Print and shaded views of the part. All mm, measured from the part's lowest x, y and z. Give positions to 0.01 mm unless a question says otherwise; leave off trailing zeros. Loops run counter-clockwise (first coordinate to the right, second up) from the corner with the lowest first, then second, coordinate; pieces in that order, holes last. Notation, with made-up numbers: (-3.75, 76) -> (16.25, 76) arc R19 ccw to (16.25, 82) -> close; hole circle Ø7 at (61.5, 52). An arc over 180 degrees is marked (long way). Answer as a JSON object with one key per item and string values. Group by question number.
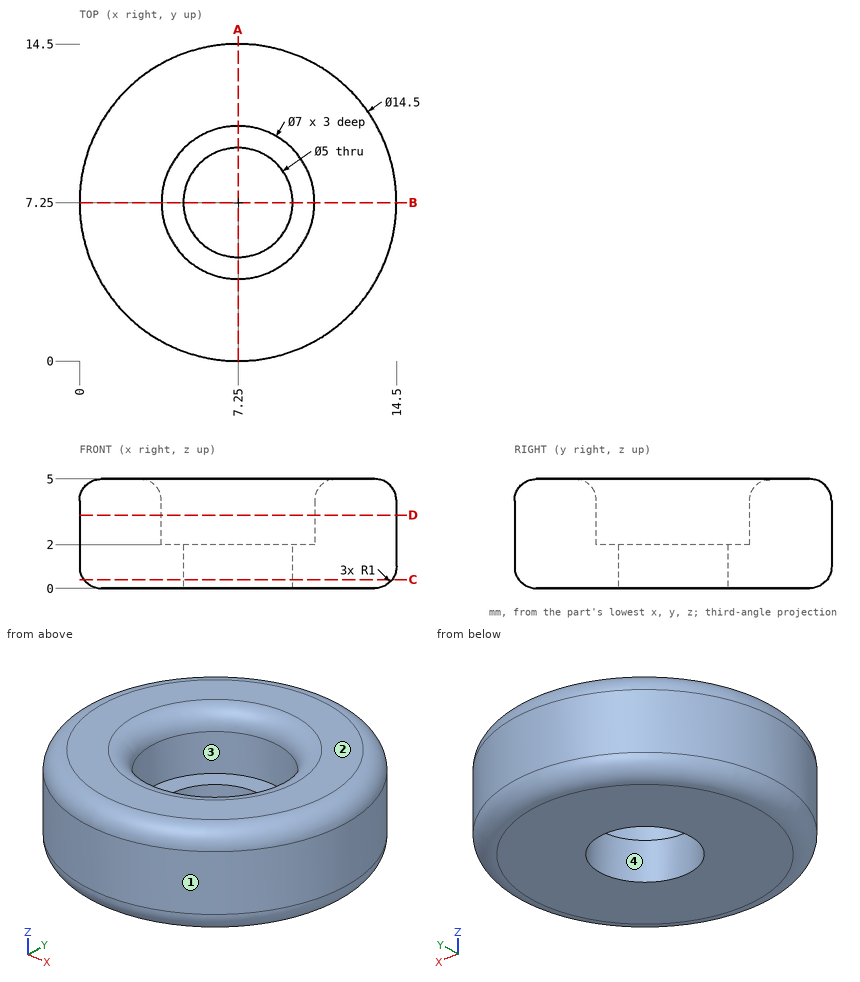
(1) Saw through at C-C on z = 0.4. List the corners of the cut face in (x, y).
(2) Saw through at A-A on x = 7.25. List the corners of the cut face in (y, z), plus the area to 3 significant figures.
(3) Probe line 1 along Y through (x, z) = (7.25, 2.95); line 2 along Z through (x, y) = (8.75, 9.75); line 3 along Y through (x, z) = (7, 0.75). List the from-to ranges inside material, lowest first. Write a range as [from, to].
(4) Saw through at D-D on z = 3.35. List the corners of the cut face in (x, y), plus the area to 3 significant figures.
(5) Pull direction Y, two halves, no side cores. Call the marked faces 1, 2, 3 and 4: pulls with the +Y half, pulls with the -Y half, needs draft (parallel to the pull), parting line crosses it, or undercut.
(6) Pin check, flat tips, straight feed: pin 1 (2 mm diameter, centred on x = 2.5, z = 2, fed in from +Y); pin 2 (3 mm diameter, centred on x = 3, z = 3.5, fed in from -Y); pin 3 (3.5 mm diameter, centred on x = 8, y = 7.5, fed in from +Z). Stop position of each tip, or through.
Calculated:
{
 "1": {"outline": "circle Ø14.1 at (7.25, 7.25); hole circle Ø5 at (7.25, 7.25)"},
 "2": {"outline": "(0, 1) arc R1 ccw to (1, 0) -> (4.75, 0) -> (4.75, 2) -> (3.75, 2) -> (3.75, 4) arc R1 ccw to (2.75, 5) -> (1, 5) arc R1 ccw to (0, 4) -> close; (9.75, 0) -> (13.5, 0) arc R1 ccw to (14.5, 1) -> (14.5, 4) arc R1 ccw to (13.5, 5) -> (11.75, 5) arc R1 ccw to (10.75, 4) -> (10.75, 2) -> (9.75, 2) -> close", "area": "40.2 mm^2"},
 "3": {"line 1": "y = [0, 3.75], [10.75, 14.5]", "line 2": "z = [0, 2]", "line 3": "y = [0.04, 4.76], [9.74, 14.46]"},
 "4": {"outline": "circle Ø14.5 at (7.25, 7.25); hole circle Ø7 at (7.25, 7.25)", "area": "127 mm^2"},
 "5": {"face 1": "parting line crosses it", "face 2": "needs draft", "face 3": "undercut", "face 4": "undercut"},
 "6": {"pin 1": "stops at y = 13.45", "pin 2": "stops at y = 0.54", "pin 3": "stops at z = 2"}
}
